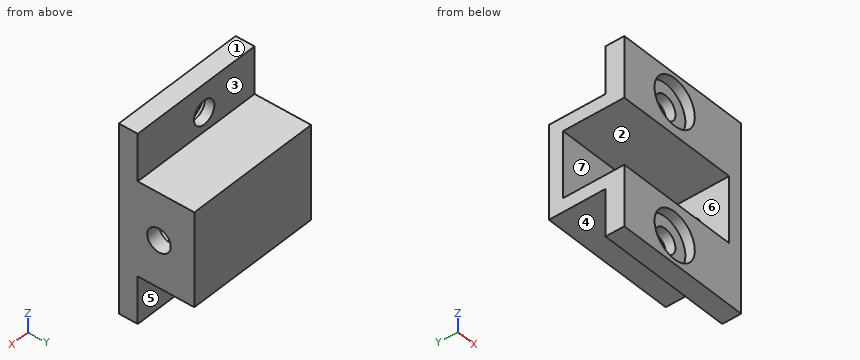
from build123d import *

# Parameters (mm, degrees)
EXTRUDE_1_DEPTH          = 6.5
EXTRUDE_2_DEPTH          = 1.5
SKETCH_3_R               = 1.25
CUT_EXTRUDE_1_DEPTH      = 21.211382931
SKETCH_4_W               = 16.5
SKETCH_4_H               = 5
EXTRUDE_3_DEPTH          = 2
SKETCH_5_R               = 1.25
CUT_EXTRUDE_2_DEPTH      = 10
SKETCH_6_R               = 2.5
CUT_EXTRUDE_3_DEPTH      = 1
CUT_EXTRUDE_4_DEPTH      = 23.14723459
CUT_EXTRUDE_4_DEPTH_BACK = 23.14723459
SKETCH_7_R               = 1.27
CUT_EXTRUDE_5_DEPTH      = 23.14723459
CUT_EXTRUDE_5_DEPTH_BACK = 23.14723459
SKETCH_8_W               = 16.5
SKETCH_8_H               = 0.229721737
SKETCH_8_H_2             = 0.3558102
CUT_EXTRUDE_6_DEPTH      = 23.758743375
CUT_EXTRUDE_6_DEPTH_BACK = 6
SKETCH_9_W               = 16.5
SKETCH_9_H               = 0.02
SKETCH_10_W              = 15.04
SKETCH_10_H              = 7.04
CUT_EXTRUDE_7_DEPTH      = 6.5
SKETCH_11_W              = 27.526079408
SKETCH_11_H              = 12.932606898
CUT_EXTRUDE_8_DEPTH      = 2


with BuildPart() as part:
    # 草图1 → 凸台-拉伸1 (new body)
    with BuildSketch(Plane(origin=(0, 0, 0), x_dir=(1, 0, 0), z_dir=(0, 1, 0))):
        Polygon((0, 1.5), (16.5, 1.5), (16.5, -8.5), (0, -8.5), (0, -7), (15, -7), (15, 0), (0, 0), align=None)
    extrude(amount=EXTRUDE_1_DEPTH)

    # 草图2 → 凸台-拉伸2 (add)
    with BuildSketch(Plane(origin=(0, 6.5, 0), x_dir=(1, 0, 0), z_dir=(0, 1, 0))):
        Polygon((0, 0), (0, -7), (0, -8.5), (16.5, -8.5), (16.5, 1.5), (0, 1.5), align=None)
    extrude(amount=EXTRUDE_2_DEPTH)

    # 草图3 → 切除-拉伸1 (cut, through all)
    with BuildSketch(Plane(origin=(16.5, 0, 0), x_dir=(0, 0, -1), z_dir=(1, 0, 0))):
        with Locations((-3.5, 4.25)):
            Circle(SKETCH_3_R)
    extrude(amount=-CUT_EXTRUDE_1_DEPTH, mode=Mode.SUBTRACT)

    # 草图4 → 凸台-拉伸3 (add)
    with BuildSketch(Plane.XZ):
        with Locations((8.25, 11)):
            Rectangle(SKETCH_4_W, SKETCH_4_H)
        with Locations((8.25, -4)):
            Rectangle(SKETCH_4_W, SKETCH_4_H)
    extrude(amount=-EXTRUDE_3_DEPTH)

    # 草图5 → 切除-拉伸2 (cut)
    with BuildSketch(Plane.XZ):
        with Locations(Location((8.25, 10.5, 0), (0, 0, 270))):
            Circle(SKETCH_5_R)
        with Locations(Location((8.25, -3.5, 0), (0, 0, 270))):
            Circle(SKETCH_5_R)
    extrude(amount=-CUT_EXTRUDE_2_DEPTH, mode=Mode.SUBTRACT)

    # 草图6 → 切除-拉伸3 (cut)
    with BuildSketch(Plane.XZ):
        with Locations(Location((8.25, 10.5, 0), (0, 0, 270))):
            Circle(SKETCH_6_R)
        with Locations(Location((8.25, -3.5, 0), (0, 0, 270))):
            Circle(SKETCH_6_R)
    extrude(amount=-CUT_EXTRUDE_3_DEPTH, mode=Mode.SUBTRACT)

    # 草图7 → 切除-拉伸4 (cut, two sides: drawn at the far end of the back side and taken through both)
    with BuildSketch(Plane(origin=(0, 2, 0), x_dir=(1, 0, 0), z_dir=(0, 1, 0)).offset(-CUT_EXTRUDE_4_DEPTH_BACK)):
        with Locations(Location((8.25, 3.5, 0), (0, 0, 270))):
            Circle(SKETCH_7_R)
        with Locations(Location((8.25, -10.5, 0), (0, 0, 270))):
            Circle(SKETCH_7_R)
    extrude(amount=CUT_EXTRUDE_4_DEPTH + CUT_EXTRUDE_4_DEPTH_BACK, mode=Mode.SUBTRACT)

    # 草图8 → 切除-拉伸5 (cut, two sides: drawn at the far end of the back side and taken through both)
    with BuildSketch(Plane(origin=(0, 2, 0), x_dir=(1, 0, 0), z_dir=(0, 1, 0)).offset(-CUT_EXTRUDE_5_DEPTH_BACK)):
        with Locations((8.25, 6.594860869)):
            Rectangle(SKETCH_8_W, SKETCH_8_H)
        with Locations((8.25, -13.6579051)):
            Rectangle(SKETCH_8_W, SKETCH_8_H_2)
    extrude(amount=CUT_EXTRUDE_5_DEPTH + CUT_EXTRUDE_5_DEPTH_BACK, mode=Mode.SUBTRACT)

    # 草图9 → 切除-拉伸6 (cut, two sides: drawn at the far end of the back side and taken through both)
    with BuildSketch(Plane(origin=(0, 8, 0), x_dir=(1, 0, 0), z_dir=(0, 1, 0)).offset(-CUT_EXTRUDE_6_DEPTH_BACK)):
        with Locations((8.25, -8.49)):
            Rectangle(SKETCH_9_W, SKETCH_9_H)
        with Locations((8.25, 1.49)):
            Rectangle(SKETCH_9_W, SKETCH_9_H)
    extrude(amount=CUT_EXTRUDE_6_DEPTH + CUT_EXTRUDE_6_DEPTH_BACK, mode=Mode.SUBTRACT)

    # 草图10 → 切除-拉伸7 (cut)
    with BuildSketch(Plane.XZ.offset(-6.5)):
        with Locations((7.5, 3.5)):
            Rectangle(SKETCH_10_W, SKETCH_10_H)
    extrude(amount=CUT_EXTRUDE_7_DEPTH, mode=Mode.SUBTRACT)

    # 草图11 → 切除-拉伸8 (cut)
    with BuildSketch(Plane.ZY):
        with Locations((5.08335855, 3.634609565)):
            Rectangle(SKETCH_11_W, SKETCH_11_H)
    extrude(amount=-CUT_EXTRUDE_8_DEPTH, mode=Mode.SUBTRACT)


solid = part.part
Model file for the job. Use its own axes, mm. Face numbers are marked on the shaded views. A direction names the side the tool comes from. Give positions to 0.01 mm unless a question says otherwise; leave off trailing zeros. Loops run counter-clockwise (first coordinate to the right, second up) from the corner with the lowest first, then second, coordinate; pieces in that order, holes last.
Item 1: Which spindle directions (+Z, -Z, +X, -X, +Y, -Y) get a long thin tool onto all of the face, cutting with end or side? Do the marked faces 1, 2 and 3. Say none if no direction does.
Check values:
face 1: +Z, +X, -X, +Y, -Y
face 2: -X, -Y
face 3: +Z, +X, -X, +Y
Item 2: Slice it at B-B (x = 8.25). Write the cut outline in (y, z).
Check values:
outline: (0, -6.48) - (2, -6.48) - (2, -4.77) - (1, -4.77) - (1, -6) - (0, -6) - close; (0, -1) - (1, -1) - (1, -2.23) - (2, -2.23) - (2, -1.48) - (8, -1.48) - (8, 8.48) - (2, 8.48) - (2, 9.23) - (1, 9.23) - (1, 8) - (0, 8) - (0, 7.02) - (6.5, 7.02) - (6.5, -0.02) - (0, -0.02) - close; (0, 13) - (1, 13) - (1, 11.77) - (2, 11.77) - (2, 13.48) - (0, 13.48) - close
Item 3: Mould opens along Z. For the marked faces 4, 5, 6 and 7 say: +Z half, -Z half, draft (parallel to the pull), parting line (faces both ways), or undercut.
Check values:
face 4: -Z half
face 5: draft
face 6: undercut
face 7: undercut
Item 4: Slice it at D-D (y = 0.75). Write the cut outline in (x, z), plus the area to 3 significant figures.
Check values:
outline: (2, -6.48) - (16.5, -6.48) - (16.5, 13.48) - (2, 13.48) - (2, 7.02) - (15.02, 7.02) - (15.02, -0.02) - (2, -0.02) - close; hole circle Ø5 at (8.25, -3.5); hole circle Ø5 at (8.25, 10.5)
area: 158 mm2
Item 5: Drop flat-ended pins along their axis: P1, Ø5.5, axis at x = 9, z = -5, coming from the +Y side; P2, Ø1.5, axis at x = 8.5, y = 5, coming from the +Z side; P3, Ø4.5, axis at x = 8.25, z = -3.5, coming from the -Y side. Give the stop position or say it passes through.
Check values:
P1: stops at y = 2
P2: stops at z = 8.48
P3: stops at y = 1
Item 6: Drill centre lines: line 1 along Z through (x, y) = (5.75, 4.5); line 2 along X through (y, z) = (0.45, -3.5); line 3 along Z through (x, y) = (8.25, 1.35). Where is each one in solid material? Low to high.
Check values:
line 1: z = -1.48 to -0.02, 7.02 to 8.48
line 2: x = 2 to 5.75, 10.75 to 16.5
line 3: z = -6.48 to -4.77, -2.23 to -0.02, 7.02 to 9.23, 11.77 to 13.48
Item 7: Slice it at A-A (y = 4.25). Write the cut outline in (x, z).
Check values:
outline: (2, -1.48) - (16.5, -1.48) - (16.5, 2.25) - (15.02, 2.25) - (15.02, -0.02) - (2, -0.02) - close; (2, 7.02) - (15.02, 7.02) - (15.02, 4.75) - (16.5, 4.75) - (16.5, 8.48) - (2, 8.48) - close
Item 8: Slice it at C-C (z = 3.5). Write the cut outline in (x, y).
Check values:
outline: (2, 6.5) - (15.02, 6.5) - (15.02, 5.5) - (16.5, 5.5) - (16.5, 8) - (2, 8) - close; (15.02, 0) - (16.5, 0) - (16.5, 3) - (15.02, 3) - close
